Read the model definition and answer for the solid it produces. Units are mm, in the model's axes. A direction names the side the tool comes from. Give positions to 0.01 mm unless a question says otherwise; leave off trailing zeros. Loops run counter-clockwise (first coordinate to the right, second up) from the corner with the lowest first, then second, coordinate; pieces in that order, holes last.
(1) Find section A-A, the plane y = 1.45. Write down the section's boundary in (x, z), then the cut area to 3 significant figures.
(2) Find section B-B, the plane y = 0.6. Write down the section's boundary in (x, z).
(3) Determine the mould class of faces 1 (the face through (-3.587, 3.678, -2.083)), 2 (the face through (0.01, 3.678, -4.148)), 3 (the face through (2.024, 2.712, -1.29)) for opening direction X: pulls with the +X half, pulls with the -X half, needs draft (parallel to the pull), parting line crosses it, or undercut.
(4) Straight lines are drawn through the part: probe 1 along X at (y, z) = (3.8, 0); probe 2 along Y at (x, z) = (-1.75, 3.25); probe 3 along Z at (x, y) = (1.75, 3.95). For each, find the intervals that lie inside material, in ascending order.
(5) Find section C-C, the plane y = 5.2. Write down the section's boundary in (x, z), then the cut area to 3 significant figures.
(6) Each of these flat-tipped pins is pushed along its axis until it touches: P1, Ø1.5, axis at y = 1.5, z = 3.5, coming from the +X side; P2, Ø1, axis at x = 3, y = 3.5, coming from the -Z side. Where does it stop, or does it pass through?
(7) Which of the six approach directions +Z, -Z, +X, -X, +Y, -Y give full straight-line access (tool end or side, diameter ignored) to faces 4 (the face through (-3.417, 4.493, -0.759)), 5 (the face through (-1.97, 1.97, -3.48))?
```python
from build123d import *

# Parameters (mm, degrees)
EXTRUDE_1_DEPTH     = 4
SKETCH_2_R          = 3.5
EXTRUDE_2_DEPTH     = 1.5
FILLET_1_R          = 0.5
SKETCH_3_R          = 2.4
CUT_EXTRUDE_1_DEPTH = 9.220908303


with BuildPart() as part:
    # 草图1 → 凸台-拉伸1 (new body)
    with BuildSketch(Plane(origin=(0, 0, 0), x_dir=(1, 0, 0), z_dir=(0, 1, 0))):
        Polygon((4, 2.309401077), (0, 4.618802154), (-4, 2.309401077), (-4, -2.309401077), (0, -4.618802154), (4, -2.309401077), align=None)
    extrude(amount=EXTRUDE_1_DEPTH)

    # 草图2 → 凸台-拉伸2 (add)
    with BuildSketch(Plane(origin=(0, 4, 0), x_dir=(1, 0, 0), z_dir=(0, 1, 0))):
        with Locations(Location((0, 0, 0), (0, 0, 270))):
            Circle(SKETCH_2_R)
    extrude(amount=EXTRUDE_2_DEPTH)

    # 圆角1
    fillet_1_edges = [part.edges().sort_by_distance(p)[0] for p in [
        (0, 5.5, -3.5),
    ]]
    fillet(fillet_1_edges, radius=FILLET_1_R)

    # 草图3 → 切除-拉伸1 (cut, through all)
    with BuildSketch(Plane.XZ):
        with Locations(Location((0, 0, 0), (0, 0, 270))):
            Circle(SKETCH_3_R)
    extrude(amount=-CUT_EXTRUDE_1_DEPTH, mode=Mode.SUBTRACT)

    # 草图4 → 切除-旋转1 (revolve, cut)
    with BuildSketch(Plane.XY):
        Polygon((4.708641342, 0), (4.708641342, 1.352262465), (4, 0), align=None)
        Polygon((4, 4), (4.708641342, 4), (4.708641342, 2.451754507), align=None)
    revolve(axis=Axis((0, 0, 0), (0, 1, 0)), mode=Mode.SUBTRACT)


solid = part.part
```
Entries:
1. outline: (-4, -2.31) - (0, -4.62) - (4, -2.31) - (4, 2.31) - (0, 4.62) - (-4, 2.31) - close; hole circle Ø4.8 at (0, 0)
1. area: 37.3 mm2
2. outline: (-4, -1.62) arc R4.31 ccw to (-3.4, -2.66) - (-0.6, -4.27) arc R4.31 ccw to (0.6, -4.27) - (3.4, -2.66) arc R4.31 ccw to (4, -1.62) - (4, 1.62) arc R4.31 ccw to (3.4, 2.66) - (0.6, 4.27) arc R4.31 ccw to (-0.6, 4.27) - (-3.4, 2.66) arc R4.31 ccw to (-4, 1.62) - close; hole circle Ø4.8 at (0, 0)
3. face 1: pulls with the -X half
3. face 2: parting line crosses it
3. face 3: undercut
4. probe 1: x = -4 to -2.4, 2.4 to 4
4. probe 2: y = 0 to 4
4. probe 3: z = -3.61 to -1.64, 1.64 to 3.61
5. outline: circle Ø6.92 at (0, 0); hole circle Ø4.8 at (0, 0)
5. area: 19.5 mm2
6. P1: stops at x = 3.24
6. P2: stops at z = -3.18
7. face 4: +Y
7. face 5: -Z, -X, +Y, -Y
